Source: CAD feature listing. Evaluate the final solid. Frame: model axes, mm. Face numbers are marked on the shaded views. Round coordinates to 2 decimals unless told otherwise and drop trailing zeros. Loops run counter-clockwise (first coordinate to the right, second up) from the corner with the lowest first, then second, coordinate; pieces in that order, holes last. Notation, with made-up numbers: (-17, 77.5) - (27, 77.5) arc R34 cw to (27, 113.5) - close; hole circle Ø1 at (30, -14). An arc over 180 degrees is marked (long way). One line per question, with ' | ' between items. Start each with the question number.
1. Cut plane D-D (x = 30.5). Return loops of the section in (y, z), then the cut area to 3 significant figures.
2. Cut plane A-A (x = -24). Return loops of the section in (y, z), then the cut area to 3 significant figures.
3. Mould query, pull axis Y, two halves, no side actions, for the marked faces 1 and 2. Classes: pulls with the +Y half, pulls with the -Y half, needs draft (parallel to the pull), parting line crosses it, or undercut.
4. Pin query (flat end, axial travel): pin 1 (3 mm diameter, centred on x = 24.5, z = -2, fed in from -Y); pin 2 (1.5 mm diameter, centred on x = 19.5, y = -4, fed in from -Z); pin 3 (0.8 mm diameter, centred on y = 34.5, z = -1.5, fed in from +X). Return the tip coordinate at first contact, or that it passes through.
5. Cut plane B-B (y = -2). Return loops of the section in (x, z).
6. Cut plane C-C (z = -2). State how many separate pieces and enclosed holes the cut face has, then the cut area to 3 significant figures.
7. Ray query, line 1 (Y direction, x = 35, z = 1.25); line 2 (Z direction, x = -6, y = 36); line 3 (Y direction, x = -24, z = -1.5). Return the intervals inside material, ascending.
```python
from build123d import *

# Parameters (mm, degrees)
SKETCH1_W           = 70
SKETCH1_H           = 50
BOSS_EXTRUDE1_DEPTH = 5
SKETCH2_W           = 2.640170668
SKETCH2_H           = 2.791037564
SKETCH2_W_2         = 2.640170669
BOSS_EXTRUDE2_DEPTH = 4
SKETCH3_W           = 7.769645109
SKETCH3_H           = 45.109201702
CUT_EXTRUDE2_DEPTH  = 2
SKETCH4_W           = 12.974552998
SKETCH4_H           = 23.007201537
BOSS_EXTRUDE3_DEPTH = 4


with BuildPart() as part:
    # Sketch1 → Boss-Extrude1 (new body)
    with BuildSketch(Plane.XY):
        with Locations((4.17218543, 13.824503311)):
            Rectangle(SKETCH1_W, SKETCH1_H)
    extrude(amount=BOSS_EXTRUDE1_DEPTH)

    # Sketch2 → Boss-Extrude2 (add)
    with BuildSketch(Plane(origin=(0, 0, 0), x_dir=(-1, 0, 0), z_dir=(0, 0, -1))):
        with Locations((-24.557996106, 34.938427472)):
            Rectangle(SKETCH2_W, SKETCH2_H)
        with Locations((-20.475121474, 34.938427472)):
            Rectangle(SKETCH2_W, SKETCH2_H)
        with Locations((-16.392246842, 34.938427472)):
            Rectangle(SKETCH2_W_2, SKETCH2_H)
        with Locations((-12.309372209, 34.938427472)):
            Rectangle(SKETCH2_W, SKETCH2_H)
        with Locations((-8.226497577, 34.938427472)):
            Rectangle(SKETCH2_W, SKETCH2_H)
        with Locations((-4.143622945, 34.938427472)):
            Rectangle(SKETCH2_W_2, SKETCH2_H)
        with Locations((-0.060748312, 34.938427472)):
            Rectangle(SKETCH2_W, SKETCH2_H)
        with Locations((4.02212632, 34.938427472)):
            Rectangle(SKETCH2_W, SKETCH2_H)
        with Locations((8.105000952, 34.938427472)):
            Rectangle(SKETCH2_W, SKETCH2_H)
        with Locations((12.187875585, 34.938427472)):
            Rectangle(SKETCH2_W, SKETCH2_H)
        with Locations((16.270750217, 34.938427472)):
            Rectangle(SKETCH2_W, SKETCH2_H)
        with Locations((20.353624849, 34.938427472)):
            Rectangle(SKETCH2_W, SKETCH2_H)
        with Locations((24.436499482, 34.938427472)):
            Rectangle(SKETCH2_W_2, SKETCH2_H)
        with Locations((28.519374114, 34.938427472)):
            Rectangle(SKETCH2_W, SKETCH2_H)
        with Locations((-25.086447815, -8.058325182)):
            Rectangle(SKETCH2_W, SKETCH2_H)
        with Locations((-21.003573182, -8.058325182)):
            Rectangle(SKETCH2_W, SKETCH2_H)
        with Locations((-16.92069855, -8.058325182)):
            Rectangle(SKETCH2_W, SKETCH2_H)
        with Locations((-12.837823918, -8.058325182)):
            Rectangle(SKETCH2_W, SKETCH2_H)
        with Locations((-8.754949286, -8.058325182)):
            Rectangle(SKETCH2_W_2, SKETCH2_H)
        with Locations((3.493674612, -8.058325182)):
            Rectangle(SKETCH2_W_2, SKETCH2_H)
        with Locations((7.576549244, -8.058325182)):
            Rectangle(SKETCH2_W, SKETCH2_H)
        with Locations((11.659423876, -8.058325182)):
            Rectangle(SKETCH2_W, SKETCH2_H)
        with Locations((15.742298508, -8.058325182)):
            Rectangle(SKETCH2_W, SKETCH2_H)
        with Locations((19.825173141, -8.058325182)):
            Rectangle(SKETCH2_W, SKETCH2_H)
        with Locations((23.908047773, -8.058325182)):
            Rectangle(SKETCH2_W, SKETCH2_H)
        with Locations((27.990922405, -8.058325182)):
            Rectangle(SKETCH2_W, SKETCH2_H)
    extrude(amount=BOSS_EXTRUDE2_DEPTH)

    # Sketch3 → Cut-Extrude2 (cut)
    with BuildSketch(Plane(origin=(0, 0, 0), x_dir=(-1, 0, 0), z_dir=(0, 0, -1))):
        with Locations((-33.251779505, 13.57301761)):
            Rectangle(SKETCH3_W, SKETCH3_H)
    extrude(amount=-CUT_EXTRUDE2_DEPTH, mode=Mode.SUBTRACT)

    # Sketch4 → Boss-Extrude3 (add)
    with BuildSketch(Plane(origin=(0, 0, 0), x_dir=(-1, 0, 0), z_dir=(0, 0, -1))):
        with Locations((16.345712334, 13.899936759)):
            Rectangle(SKETCH4_W, SKETCH4_H)
    extrude(amount=BOSS_EXTRUDE3_DEPTH)


solid = part.part
```
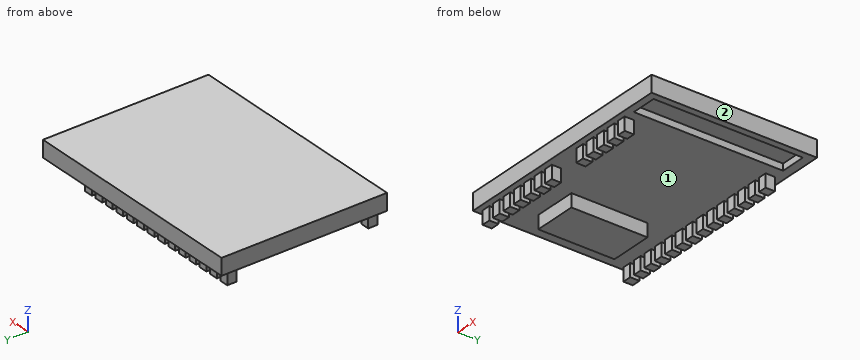
Answers follow:
1) outline: (-11.18, 0) - (-8.98, 0) - (-8.98, 2) - (36.13, 2) - (36.13, 0) - (38.82, 0) - (38.82, 5) - (-11.18, 5) - close | area: 160 mm2
2) outline: (-11.18, 0) - (-9.45, 0) - (-9.45, -4) - (-6.66, -4) - (-6.66, 0) - (33.54, 0) - (33.54, -4) - (36.33, -4) - (36.33, 0) - (38.82, 0) - (38.82, 5) - (-11.18, 5) - close | area: 272 mm2
3) face 1: undercut | face 2: needs draft
4) pin 1: stops at y = -9.45 | pin 2: stops at z = 0 | pin 3: stops at x = 25.88
5) outline: (-30.83, 0) - (29.37, 0) - (29.37, 2) - (37.14, 2) - (37.14, 0) - (39.17, 0) - (39.17, 5) - (-30.83, 5) - close
6) separate pieces: 27 | enclosed holes: 0 | area: 490 mm2
7) line 1: y = -11.18 to -8.98, 36.13 to 38.82 | line 2: z = 0 to 5 | line 3: y = -9.45 to -6.66, 33.54 to 36.33
